```python
from build123d import *

# Parameters (mm, degrees)
SKETCH2_R           = 125
BOSS_EXTRUDE1_DEPTH = 3
CUT_EXTRUDE1_DEPTH  = 3
SKETCH4_R           = 1.65
SKETCH4_R_2         = 5
CUT_EXTRUDE2_DEPTH  = 10


with BuildPart() as part:
    # Sketch2 → Boss-Extrude1 (new body)
    with BuildSketch(Plane(origin=(0, 0, 0), x_dir=(1, 0, 0), z_dir=(0, 1, 0))):
        with Locations((-17.80765369, -0.854894607)):
            Circle(SKETCH2_R)
    extrude(amount=BOSS_EXTRUDE1_DEPTH)

    # Sketch3 → Cut-Extrude1 (cut)
    with BuildSketch(Plane.XZ):
        Polygon((-735.289651923, 45.854894607), (-134.426691587, 45.854894607), (98.811384207, 45.854894607), (699.674344543, 45.854894607), (699.674344543, 1247.580815278), (-735.289651923, 1247.580815278), align=None)
    extrude(amount=-CUT_EXTRUDE1_DEPTH, mode=Mode.SUBTRACT)

    # Sketch4 → Cut-Extrude2 (cut)
    with BuildSketch(Plane(origin=(0, 0, 0), x_dir=(-1, 0, 0), z_dir=(0, -1, 0))):
        with Locations((117.80765369, 54.145105393)):
            Circle(SKETCH4_R)
        with Locations((117.881226527, 23.145192699)):
            Circle(SKETCH4_R)
        with Locations((103.80765369, 54.145105393)):
            Circle(SKETCH4_R)
        with Locations((103.80765369, 23.145105393)):
            Circle(SKETCH4_R)
        with Locations((-68.19234631, 54.267083079)):
            Circle(SKETCH4_R)
        with Locations((-82.19234631, 54.267083079)):
            Circle(SKETCH4_R)
        with Locations((-82.19234631, 23.267083079)):
            Circle(SKETCH4_R)
        with Locations((-68.19234631, 23.267083079)):
            Circle(SKETCH4_R)
        with Locations((122.80765369, -35.854894607)):
            Circle(SKETCH4_R_2)
        with Locations((-87.19234631, -35.854894607)):
            Circle(SKETCH4_R_2)
        Polygon((124.881226527, 63.645105393), (124.881226527, 13.645105393), (141.357501756, 13.645105393), (159.377606719, 40.481299306), align=None)
        Polygon((-89.19234631, 63.767083079), (-89.19234631, 13.767083079), (-106.334191667, 13.767083079), (-114.079843912, 54.596315864), align=None)
    extrude(amount=-CUT_EXTRUDE2_DEPTH, mode=Mode.SUBTRACT)


solid = part.part
```
The model under review builds one solid part; all positions refer to its coordinate system, in mm. Coordinates: 2 decimals unless noted, no trailing zeros. Write each loop counter-clockwise with the first axis right and the second up, starting at its lowest first coordinate (ties: lowest second). Pieces come first, ordered by that corner, then holes.
1) We need section B-B on z = -94. State the section outline as (x, y) points, then the cut area to 3 significant figures.
2) Clearance check with flat-ended pins moving along their axes: pin 1 Ø1.5 at (x, y) = (50, 2) entering from -Z; pin 2 Ø1.5 at (x, y) = (-130.5, 1.5) entering from -Z; pin 3 Ø2.5 at (x, z) = (-117.81, -54.15) entering from -Y; pin 4 Ø1 at (y, z) = (2, 10.5) entering from -X. State where each tip first meets the part, or that it passes through.
3) We need section A-A on y = 0.65. Count the separate pieces of the cut face and the enclosed holes in it, then the cut area to 3 significant figures.
4) We need section C-C on x = -68. State the section outline as (y, z) points, then the cut area to 3 significant figures.
5) To check wall thickness, follow probe 1 along X at (y, z) = (2.2, -54); probe 2 along X at (y, z) = (1.9, -23.5); probe 3 along Z at (x, y) = (69, 1.8). State the ranges of each line that lie inside material, in increasing order.
6) The part is to be moulded in two halves that separate along X. For faces 1 (the face through (-141.916, 1.479, 15.755)), 2 (the face through (-127.426, 1.479, 37.77)), 3 (the face through (-16.08, 1.479, -124.133)), say which applies: pulls with the +X half, pulls with the -X half, needs draft (parallel to the pull), parting line crosses it, or undercut.
Answer list:
1. outline: (-99.22, 0) - (63.6, 0) - (63.6, 3) - (-99.22, 3) - close
1. area: 488 mm2
2. pin 1: stops at z = -104.64
2. pin 2: stops at z = -13.65
2. pin 3: passes through
2. pin 4: stops at x = -142.47
3. separate pieces: 1
3. enclosed holes: 10
3. area: 34,300 mm2
4. outline: (0, -113.63) - (3, -113.63) - (3, 45.85) - (0, 45.85) - close
4. area: 478 mm2
5. probe 1: x = -124.88 to -119.45, -116.16 to -105.45, -102.16 to 66.56, 69.82 to 80.56, 83.82 to 89.19
5. probe 2: x = -124.88 to -119.49, -116.27 to -105.42, -102.2 to 66.56, 69.83 to 80.56, 83.83 to 89.19
5. probe 3: z = -89.09 to -55.71, -52.83 to -24.71, -21.83 to 45.85
6. face 1: pulls with the -X half
6. face 2: undercut
6. face 3: parting line crosses it
